```python
from build123d import *

# Parameters (mm, degrees)
F0_R     = 7
F0_R_2   = 3.75
F1_DEPTH = 31
F0_R_3   = 9
F2_DEPTH = 3
F3_DEPTH = 3
F4_DEPTH = 3
F5_DEPTH = 35


with BuildPart() as f1:
    # F0 (on Front) → F1 (new body)
    with BuildSketch(Plane.XZ):
        Circle(F0_R)
        Circle(F0_R_2, mode=Mode.SUBTRACT)
    extrude(amount=F1_DEPTH)

    # F0 (on Front) → F2 (join)
    with BuildSketch(Plane.XZ):
        Circle(F0_R_3)
        Circle(F0_R, mode=Mode.SUBTRACT)
    extrude(amount=F2_DEPTH)

    # F0 (on Front) → F3 (join)
    with BuildSketch(Plane.XZ):
        Circle(F0_R)
        Circle(F0_R_2, mode=Mode.SUBTRACT)
    extrude(amount=-F3_DEPTH)

    # F0 (on Front) → F4 (join)
    with BuildSketch(Plane.XZ):
        Circle(F0_R_2)
    extrude(amount=-F4_DEPTH)

    # F0 (on Front) → F5 (join)
    with BuildSketch(Plane.XZ):
        Circle(F0_R_2)
    extrude(amount=F5_DEPTH)


solid = f1.part
```
Source: CAD feature listing. Evaluate the final solid. Frame: model axes, mm. A direction names the side the tool comes from. Round coordinates to 2 decimals unless told otherwise and drop trailing zeros. Loops run counter-clockwise (first coordinate to the right, second up) from the corner with the lowest first, then second, coordinate; pieces in that order, holes last. Notation, with made-up numbers: M 47,43.25 L 63,43.25 A27 cw 63,77.25 Z; hole C -15.5,-22 d2. An arc over 180 degrees is marked long. Use a Markdown table: item, result. Add a question column.
1. Section query D-D on z = -6.5. Return the cut outline in (x, y).
2. Section query C-C on y = -26. Return the cut outline in (x, z).
3. Section query A-A on x = 0. Return the cut outline in (y, z).
4. Section query B-B on z = 0. Return the cut outline in (x, y), then the cut area to 3 significant figures.
5. Contact query for flat-ended pins moving along their axis: P1, Ø2, axis at y = -26.5, z = 0.5, coming from the -X side; P2, Ø1.5, axis at x = -6, y = -26.5, coming from the +Z side; P3, Ø1.5, axis at x = 0, y = -17, coming from the -Z side. Output: stop coordinate, or through.
6. Reachability of faces 1 (the flat face through (0, -35, 0)), 2 (the flat face through (0, 0, -7.3)), 3 (the flat face through (3, -31, -3)) from +Z, -Z, +X, -X, +Y, -Y: full face, straight path, thin tool, end or side. Return the list, or none.
7. Line query: line 1 (Y direction, x = 8.25, z = -3.25); line 2 (Y direction, x = -5.5, z = -1.25); line 3 (Z direction, x = -5, y = -15.5). Output: solid intervals per line, ascending.
Reported:
| question | item | result |
|---|---|---|
| 1 | outline | M -6.22,-3 L -2.6,-3 L -2.6,-31 L 2.6,-31 L 2.6,-3 L 6.22,-3 L 6.22,0 L 2.6,0 L 2.6,3 L -2.6,3 L -2.6,0 L -6.22,0 Z |
| 2 | outline | C 0,0 d14 |
| 3 | outline | M -35,-3.75 L -31,-3.75 L -31,-7 L -3,-7 L -3,-9 L 0,-9 L 0,-7 L 3,-7 L 3,7 L 0,7 L 0,9 L -3,9 L -3,7 L -31,7 L -31,3.75 L -35,3.75 Z |
| 4 | outline | M -9,-3 L -7,-3 L -7,-31 L -3.75,-31 L -3.75,-35 L 3.75,-35 L 3.75,-31 L 7,-31 L 7,-3 L 9,-3 L 9,0 L 7,0 L 7,3 L -7,3 L -7,0 L -9,0 Z |
| 4 | area | 518 mm² |
| 5 | P1 | stops at x = -7 |
| 5 | P2 | stops at z = 4.63 |
| 5 | P3 | stops at z = -7 |
| 6 | face 1 | +Z, -Z, +X, -X, -Y |
| 6 | face 2 | +Y |
| 6 | face 3 | -Y |
| 7 | line 1 | y = -3 to 0 |
| 7 | line 2 | y = -31 to 3 |
| 7 | line 3 | z = -4.9 to 4.9 |
